Part model, mm, in its own coordinate system. A direction names the side the tool comes from. Coordinates: 2 decimals unless noted, no trailing zeros. Order: outer loops, then holes, each group sorted by start corner. A loop starts at its lowest first (then second) coordinate and runs counter-clockwise, first axis right, second up. Notation, with made-up numbers: (-1, 76.25) - (29, 76.25) arc R10 cw to (29, 80.25) - close; hole circle Ø10 at (-24.75, 0.5). An arc over 180 degrees is marked (long way). Use a Markdown table: item, result. Add a question column.
1) Wall check: L1, parallel to X at y = -106.5, z = 72; L2, parallel to X at y = -51.5, z = 22.5; L3, parallel to Z at x = -32, y = -19. Give the ranges that are in metal, low to high. Write a range as [from, to].
2) Two-plate mould, pull along Z, no slides. Class faces 6 (the face through (-11.504, -63.375, 10.819)), 7 (the face through (-35, -62, 100)), 8 (the face through (-27, 0, 53)), 9 (the face through (-30, -62, 55)): +Z half, -Z half, draft (parallel to the pull), parting line (faces both ways), or undercut.
3) Tool access for faces 1 (the face through (-50.463, -98.176, 4.683)), 2 (the face through (-20, -62, 69)), 3 (the face through (-49, -63, 148)), 4 (the face through (6, -103, -4)), 5 (the face through (-10.36, -21.87, -2.76)): list every direction of +Z, -Z, +X, -X, +Y, -Y with a clear straight run to the whole face (end or side of a thin tool).
4) Saw through at B-B on z = 81. List the corners of the cut face in (x, y), then the cut area to 3 significant figures.
5) Saw through at C-C on z = 30. List the corners of the cut face in (x, y), then the cut area to 3 significant figures.
6) Drop flat-ended pins along their axis: P1, Ø7, axis at y = -85.5, z = 5, coming from the -X side; P2, Ø11, axis at x = -33, y = -41.5, coming from the -Z side; P3, Ø6, axis at y = -45.5, z = 7, coming from the +X side. Give the stop position or say it passes through.
7) Saw through at A-A on x = -36. List the corners of the cut face in (y, z).
```python
from build123d import *

# Parameters (mm, degrees)
F0_W     = 10
F0_H     = 69.7555384352
F1_DEPTH = 125
F2_R     = 1
F3_R     = 4.99999
F5_R     = 5
F6_R     = 5
F8_R     = 27.5
F9_DEPTH = 128.1414455964


# Not quite as in the source:
# - two fillets or chamfers of one size are made in one step
# - a fillet or chamfer is up to 0.001 mm smaller than in the source, because OpenCascade refuses the exact size


with BuildPart() as f1:
    # F0 (on Front) → F1 (new body)
    with BuildSketch(Plane.XZ):
        Polygon((-50, 150), (-50, 20), (-80, 0), (-51.7332726626, -2.9754449829), (-50.8957943865, 4.9805986405), (-40, 12.2444615648), (-30, 12.2444615648), (-10, 12.2444615648), (-10, 10), (-10, 0.6757781788), (-10.8374782761, -7.2802654446), (15, -10), (0, 0), (0, 45), (-10, 45), (-10, 20), (-20, 20), (-20, 125), (-30, 125), (-30, 100), (-40, 100), (-40, 150), align=None)
        with Locations((-35, 55.1222307824)):
            Rectangle(F0_W, F0_H, mode=Mode.SUBTRACT)
    extrude(amount=F1_DEPTH)

    # F2
    f2_edges = [f1.edges().sort_by_distance(p)[0] for p in [
        (-80, -62.5, 0),
        (-10.837478, -62.5, -7.280265),
        (15, -62.5, -10),
        (-51.733273, -62.5, -2.975445),
        (0, -62.5, 0),
    ]]
    fillet(f2_edges, radius=F2_R)

    # F3 (radius 5 in the source; OpenCascade refuses exactly that, so slightly less here)
    f3_edges = [f1.edges().sort_by_distance(p)[0] for p in [
        (0, -62.5, 45),
        (-10, -62.5, 45),
        (-20, -62.5, 125),
        (-30, -62.5, 125),
        (-40, -62.5, 150),
        (-50, -62.5, 150),
    ]]
    fillet(f3_edges, radius=F3_R)

    # F5
    f5_edges = [f1.edges().sort_by_distance(p)[0] for p in [
        (-50.895794, -62.5, 4.980599),
        (-40, -62.5, 12.244462),
        (-10, -62.5, 12.244462),
    ]]
    fillet(f5_edges, radius=F5_R)

    # F6
    f6_edges = [f1.edges().sort_by_distance(p)[0] for p in [
        (-50, -62.5, 20),
    ]]
    fillet(f6_edges, radius=F6_R)

    # F8 (on offset) → F9 (cut, through all)
    with BuildSketch(Plane.YZ.offset(50)):
        with Locations((-62.5, -20)):
            Circle(F8_R)
    extrude(amount=-F9_DEPTH, mode=Mode.SUBTRACT)


solid = f1.part
```
Results are:
| question | item | result |
|---|---|---|
| 1 | L1 | [-50, -40], [-30, -20] |
| 1 | L2 | [-50, -40], [-30, -20], [-10, 0] |
| 1 | L3 | [12.24, 20.24], [90, 100] |
| 2 | face 6 | undercut |
| 2 | face 7 | +Z half |
| 2 | face 8 | draft |
| 2 | face 9 | undercut |
| 3 | face 1 | -Z, +Y, -Y |
| 3 | face 2 | +Z, +Y, -Y |
| 3 | face 3 | +Z, -X, +Y, -Y |
| 3 | face 4 | +Z, +X, +Y, -Y |
| 3 | face 5 | +Y, -Y |
| 4 | outline | (-50, -125) - (-40, -125) - (-40, 0) - (-50, 0) - close; (-30, -125) - (-20, -125) - (-20, 0) - (-30, 0) - close |
| 4 | area | 2,500 mm2 |
| 5 | outline | (-50, -125) - (-40, -125) - (-40, 0) - (-50, 0) - close; (-30, -125) - (-20, -125) - (-20, 0) - (-30, 0) - close; (-10, -125) - (0, -125) - (0, 0) - (-10, 0) - close |
| 5 | area | 3,750 mm2 |
| 6 | P1 | x = -77.75 |
| 6 | P2 | z = 12.24 |
| 6 | P3 | x = 0 |
| 7 | outline | (-125, 12.24) - (0, 12.24) - (0, 20.24) - (-125, 20.24) - close; (-125, 90) - (0, 90) - (0, 100) - (-125, 100) - close |
